Can you work these out from the model? Positions are in its coordinate system, mm. A direction names the side the tool comes from. Give positions to 0.01 mm unless a question says otherwise; leave off trailing zeros. Order: outer loops, then holes, each group sorted by start corner. A loop starts at its lowest first (then second) coordinate and runs counter-clockwise, first axis right, second up. Notation, with made-up numbers: (-13.75, 82) -> (6.25, 82) arc R21 cw to (6.25, 118) -> close; hole circle Ø3 at (-21, 28). An arc over 180 degrees is marked (long way). Answer as CSV lines item,"result".
```python
from build123d import *

# Parameters (mm, degrees)
BOSS_EXTRUDE1_DEPTH     = 6
SKETCH2_R               = 4
SKETCH2_R_2             = 15
CUT_EXTRUDE1_DEPTH      = 313.353853826
CROQUIS2_W              = 97
CROQUIS2_H              = 0.3
CORTAR_EXTRUIR1_DEPTH   = 10
CORTAR_EXTRUIR2_DEPTH   = 10
CROQUIS4_R              = 4
CORTAR_EXTRUIR3_DEPTH   = 6
SALIENTE_EXTRUIR2_DEPTH = 6
CROQUIS7_W              = 0.3
CROQUIS7_H              = 222.05
CORTAR_EXTRUIR4_DEPTH   = 6
CROQUIS8_W              = 25
CROQUIS8_H              = 12
CORTAR_EXTRUIR5_DEPTH   = 6
SALIENTE_EXTRUIR3_DEPTH = 10
CORTAR_EXTRUIR6_DEPTH   = 10
SALIENTE_EXTRUIR4_DEPTH = 16
CROQUIS12_W             = 25.313873874
CROQUIS12_H             = 10
CORTAR_EXTRUIR7_DEPTH   = 67
CROQUIS13_R             = 4
CORTAR_EXTRUIR8_DEPTH   = 10
SALIENTE_EXTRUIR5_DEPTH = 6
CROQUIS15_R             = 4
CORTAR_EXTRUIR9_DEPTH   = 10
SALIENTE_EXTRUIR7_DEPTH = 6
CROQUIS18_R             = 4
CORTAR_EXTRUIR10_DEPTH  = 6
SALIENTE_EXTRUIR8_DEPTH = 6


with BuildPart() as part:
    # Sketch1 → Boss-Extrude1 (new body)
    with BuildSketch(Plane.XY):
        Polygon((0, 0), (143.3, 0), (143.3, 8.3), (173.3, 8.3), (173.3, 60), (60, 259.8), (0, 259.8), align=None)
    extrude(amount=BOSS_EXTRUDE1_DEPTH)

    # Sketch2 → Cut-Extrude1 (cut, through all)
    with BuildSketch(Plane.XY.offset(6)):
        with Locations((158.3, 36.3)):
            Circle(SKETCH2_R)
        with Locations((37.8, 244.8)):
            Circle(SKETCH2_R)
        with Locations((37.8, 125)):
            Circle(SKETCH2_R)
        with Locations((80, 43.8)):
            Circle(SKETCH2_R)
        with Locations((70, 85)):
            Circle(SKETCH2_R_2)
        Polygon((46.3, 0), (46.3, 19), (19, 46.3), (0, 46.3), (0, 0), align=None)
    extrude(amount=-CUT_EXTRUDE1_DEPTH, mode=Mode.SUBTRACT)

    # Croquis2 → Cortar-Extruir1 (cut)
    with BuildSketch(Plane.XY.offset(6)):
        with Locations((94.8, 0.15)):
            Rectangle(CROQUIS2_W, CROQUIS2_H)
    extrude(amount=-CORTAR_EXTRUIR1_DEPTH, mode=Mode.SUBTRACT)

    # Croquis3 → Cortar-Extruir2 (cut)
    with BuildSketch(Plane.XY.offset(6)):
        Polygon((46.3, 19), (19, 46.3), (27, 46.3), (46.3, 27), align=None)
    extrude(amount=-CORTAR_EXTRUIR2_DEPTH, mode=Mode.SUBTRACT)

    # Croquis4 → Cortar-Extruir3 (cut)
    with BuildSketch(Plane.XY.offset(6)):
        with Locations((80, 36.3)):
            Circle(CROQUIS4_R)
        with Locations((80, 43.8)):
            Circle(CROQUIS4_R)
    extrude(amount=-CORTAR_EXTRUIR3_DEPTH, mode=Mode.SUBTRACT)

    # Croquis6 → Saliente-Extruir2 (add)
    with BuildSketch(Plane.XY.offset(6)):
        with BuildLine():
            ThreePointArc((81.391941091, 40.05), (83.283882181, 41.516117819), (84, 43.8))
            ThreePointArc((84, 43.8), (77.716117819, 47.083882181), (78.608058909, 40.05))
            ThreePointArc((78.608058909, 40.05), (80, 40.3), (81.391941091, 40.05))
        make_face()
    extrude(amount=-SALIENTE_EXTRUIR2_DEPTH)

    # Croquis7 → Cortar-Extruir4 (cut)
    with BuildSketch(Plane.XY.offset(6)):
        with Locations((0.15, 148.775)):
            Rectangle(CROQUIS7_W, CROQUIS7_H)
    extrude(amount=-CORTAR_EXTRUIR4_DEPTH, mode=Mode.SUBTRACT)

    # Croquis8 → Cortar-Extruir5 (cut)
    with BuildSketch(Plane.XY.offset(6)):
        with Locations((12.8, 159.05)):
            Rectangle(CROQUIS8_W, CROQUIS8_H)
    extrude(amount=-CORTAR_EXTRUIR5_DEPTH, mode=Mode.SUBTRACT)

    # Croquis10 → Cortar-Extruir6 (cut)
    with BuildSketch(Plane.XY.offset(6)):
        Polygon((147.986126126, 104.64), (146.286126126, 104.64), (146.286126126, 107.63788173), align=None)
    extrude(amount=-CORTAR_EXTRUIR6_DEPTH, mode=Mode.SUBTRACT)



with BuildPart() as body_2:
    # Croquis9 → Saliente-Extruir3 (new body)
    with BuildSketch(Plane.XY.offset(6)):
        Polygon((147.986126126, 104.64), (173.3, 60), (173.3, 104.64), align=None)
    extrude(amount=SALIENTE_EXTRUIR3_DEPTH)


with BuildPart() as part_1:
    add(part.part)

    add(body_2.part)  # Saliente-Extruir4 merges body 2
    # Croquis11 → Saliente-Extruir4 (add)
    with BuildSketch(Plane.XY.offset(16)):
        Polygon((173.3, 60), (173.3, 104.64), (147.986126126, 104.64), align=None)
    extrude(amount=-SALIENTE_EXTRUIR4_DEPTH)

    # Croquis12 → Cortar-Extruir7 (cut)
    with BuildSketch(Plane(origin=(0, 104.64, 0), x_dir=(1, 0, 0), z_dir=(0, 1, 0))):
        with Locations((160.643063063, -11)):
            Rectangle(CROQUIS12_W, CROQUIS12_H)
    extrude(amount=-CORTAR_EXTRUIR7_DEPTH, mode=Mode.SUBTRACT)

    # Croquis13 → Cortar-Extruir8 (cut)
    with BuildSketch(Plane.XY.offset(6)):
        with Locations((80, 41.8)):
            Circle(CROQUIS13_R)
    extrude(amount=-CORTAR_EXTRUIR8_DEPTH, mode=Mode.SUBTRACT)

    # Croquis14 → Saliente-Extruir5 (add)
    with BuildSketch(Plane.XY.offset(6)):
        with BuildLine():
            ThreePointArc((82.90473751, 39.05), (80, 37.8), (77.09526249, 39.05))
            ThreePointArc((77.09526249, 39.05), (78.519957777, 32.5838898), (84, 36.3))
            ThreePointArc((84, 36.3), (83.7161102, 37.780042223), (82.90473751, 39.05))
        make_face()
    extrude(amount=-SALIENTE_EXTRUIR5_DEPTH)

    # Croquis15 → Cortar-Extruir9 (cut)
    with BuildSketch(Plane.XY.offset(6)):
        with Locations((80, 47.3)):
            Circle(CROQUIS15_R)
    extrude(amount=-CORTAR_EXTRUIR9_DEPTH, mode=Mode.SUBTRACT)

    # Croquis16 → Saliente-Extruir7 (add)
    with BuildSketch(Plane.XY.offset(6)):
        with BuildLine():
            ThreePointArc((77.09526249, 44.55), (78.519957777, 38.0838898), (84, 41.8))
            ThreePointArc((84, 41.8), (83.7161102, 43.280042223), (82.90473751, 44.55))
            ThreePointArc((82.90473751, 44.55), (80, 43.3), (77.09526249, 44.55))
        make_face()
    extrude(amount=-SALIENTE_EXTRUIR7_DEPTH)

    # Croquis18 → Cortar-Extruir10 (cut)
    with BuildSketch(Plane.XY.offset(6)):
        with Locations((80, 41.8)):
            Circle(CROQUIS18_R)
    extrude(amount=-CORTAR_EXTRUIR10_DEPTH, mode=Mode.SUBTRACT)

    # Croquis19 → Saliente-Extruir8 (add)
    with BuildSketch(Plane.XY.offset(6)):
        with BuildLine():
            ThreePointArc((82.90473751, 44.55), (83.7161102, 45.819957777), (84, 47.3))
            ThreePointArc((84, 47.3), (78.519957777, 51.0161102), (77.09526249, 44.55))
            ThreePointArc((77.09526249, 44.55), (80, 45.8), (82.90473751, 44.55))
        make_face()
    extrude(amount=-SALIENTE_EXTRUIR8_DEPTH)


solid = part_1.part
```
Item 1: For faces 5 (the flat face through (46.3, 13, 3)), 6 (the flat face through (158, 8.3, 3)), 7 (the flat face through (160, 104.64, 3)), which set-ups out of +Z, -Z, +X, -X, +Y, -Y let a thin tool reach every point of the face, with its end or its side?
Numbers:
face 5,"+Z, -Z, -X, -Y"
face 6,"+Z, -Z, +X, -Y"
face 7,"+Z, -Z, +X, +Y"
Item 2: Imagine slicing it at C-C, the plane x = 80. Please give me the cut outline in (y, z), then the cut area to 3 significant figures.
Numbers:
outline,"(0.3, 0) -> (37.8, 0) -> (37.8, 6) -> (0.3, 6) -> close; (45.8, 0) -> (73.82, 0) -> (73.82, 6) -> (45.8, 6) -> close; (96.18, 0) -> (224.53, 0) -> (224.53, 6) -> (96.18, 6) -> close"
area,"1,160 mm²"
Item 3: We'd pull the mould along Y, two halves only. Please class faces 1 (the flat face through (143.3, 4, 3)), 2 (the flat face through (13, 165.05, 3)), 3 (the cylindrical face through (39.95, 248.173, 3.042)), 4 (the flat face through (103.75, 182.65, 2.96)): released by +Y, released by -Y, zero draft, split by the parting line, or undercut.
Numbers:
face 1,"zero draft"
face 2,"undercut"
face 3,"undercut"
face 4,"released by +Y"
Item 4: Please list where these lines run through material, in increasing order: line 1 along Y through (x, z) = (158.3, 3.2); line 2 along Y through (x, z) = (37.8, 3); line 3 along Y through (x, z) = (157, 3.25).
Numbers:
line 1,"y = 8.3 to 32.3, 40.3 to 104.64"
line 2,"y = 35.5 to 121, 129 to 240.8, 248.8 to 259.8"
line 3,"y = 8.3 to 32.52, 40.08 to 104.64"
Item 5: Imagine slicing it at D-D, the plane x = 159. Please give me the cut outline in (y, z), then the cut area to 3 significant figures.
Numbers:
outline,"(8.3, 0) -> (32.36, 0) -> (32.36, 6) -> (8.3, 6) -> close; (40.24, 0) -> (104.64, 0) -> (104.64, 6) -> (40.24, 6) -> close"
area,"531 mm²"
Item 6: For pin 1 (10.5 mm diameter, centred on x = 37.8, y = 244.8, fed in from -Z); pin 2 (3 mm diameter, centred on x = 17, z = 2.5, fed in from -Y); pin 3 (3 mm diameter, centred on x = 165.5, z = 1.5, fed in from +Y); pin 4 (1.5 mm diameter, centred on y = 106.5, z = 3, fed in from +X), each with a flat end and sliding along its axis, tell me the tip position at first contact or that it passes through.
Numbers:
pin 1,"stops at z = 0"
pin 2,"stops at y = 46.3"
pin 3,"stops at y = 104.64"
pin 4,"stops at x = 146.29"
Item 7: Imagine slicing it at B-B, the plane z = 3.25. Please give me the cut outline in (x, y).
Numbers:
outline,"(0.3, 46.3) -> (27, 46.3) -> (46.3, 27) -> (46.3, 0.3) -> (143.3, 0.3) -> (143.3, 8.3) -> (173.3, 8.3) -> (173.3, 104.64) -> (146.29, 104.64) -> (146.29, 107.64) -> (60, 259.8) -> (0.3, 259.8) -> (0.3, 165.05) -> (25.3, 165.05) -> (25.3, 153.05) -> (0.3, 153.05) -> close; hole circle Ø8 at (37.8, 125); hole circle Ø8 at (37.8, 244.8); hole circle Ø30 at (70, 85); hole circle Ø8 at (80, 41.8); hole circle Ø8 at (158.3, 36.3)"
Item 8: Imagine slicing it at A-A, the plane y = 85. Please give me the cut outline in (x, z).
Numbers:
outline,"(0.3, 0) -> (55, 0) -> (55, 6) -> (0.3, 6) -> close; (85, 0) -> (173.3, 0) -> (173.3, 6) -> (85, 6) -> close"
